Build history of the part. All positions in model axes, mm. Face numbers are marked on the shaded views. A direction names the side the tool comes from. Coordinates: 2 decimals unless noted, no trailing zeros. Order: outer loops, then holes, each group sorted by start corner. A loop starts at its lowest first (then second) coordinate and runs counter-clockwise, first axis right, second up. Notation, with made-up numbers: M 41.5,76 L 72.5,76 A27 cw 72.5,97 Z; hole C 60.5,-29 d10. An arc over 180 degrees is marked long. Write item = value, one per line. Start each with the question number.
Q1. Band-saw the part on D-D on x = 41.5. Write the cut outline in (y, z).
Q2. Band-saw the part on A-A on y = 18. Write the cut outline in (x, z).
Q3. Pull direction X, two halves, no side cores. Call the marked faces 1, 2, 3 and 4: released by +X, released by -X, zero draft, split by the parting line, or undercut.
Q4. Pin check, flat tips, straight feed: P1, Ø3, axis at x = 68.5, z = 4, coming from the +Y side; P2, Ø3.5, axis at x = 66.91, y = 18, coming from the +Z side; P3, Ø1, axis at x = 72, z = 9, coming from the -Y side; P4, Ø1.6, axis at y = 2.5, z = 4, coming from the +X side. Stop position of each tip, or through.
Q5. 3-axis set-ups, long thin cutter, end or side, ignore diameter. For the marked faces 5 and 6: which of +Z, -Z, +X, -X, +Y, -Y reach the whole face in a straight line?
Q6. Band-saw the part on B-B on x = 71.5. Write the cut outline in (y, z).
Q7. Drill centre lines: probe 1 along X at (y, z) = (17, 2.25); probe 2 along X at (y, z) = (40, 8.5); probe 3 along X at (y, z) = (19.5, 1.5). Where is each one in solid material? Low to high.
Q8. Band-saw the part on C-C on z = 4.25. State how many separate pieces and enclosed holes the cut face has, plus the area to 3 significant figures.
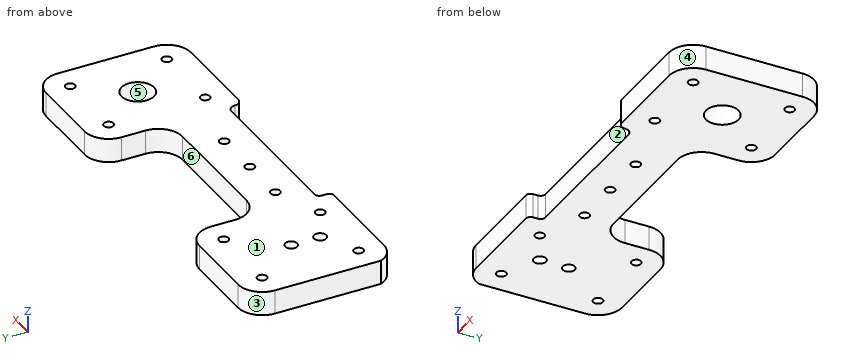
```python
from build123d import *

# Parameters (mm, degrees)
MODEL_R             = 2
MODEL_R_2           = 2.5
MODEL_R_3           = 6.75
MODEL_R_4           = 2.55
BOSS_EXTRUDE1_DEPTH = 10


with BuildPart() as part:
    # Model → Boss-Extrude1 (new body)
    with BuildSketch(Plane.XY):
        with BuildLine():
            Line((-13.089430894, 50), (-13.089430894, 6))
            ThreePointArc((-13.089430894, 6), (-9.401505079, 1.633399735), (-3.924279504, 0))
            Line((-3.924279504, 0), (34.910569106, 0))
            ThreePointArc((34.910569106, 0), (36.324782668, 0.585786438), (36.910569106, 2))
            Line((36.910569106, 2), (36.910569106, 4))
            ThreePointArc((36.910569106, 4), (37.496355543, 5.414213562), (38.910569106, 6))
            Line((38.910569106, 6), (103.910569106, 6))
            ThreePointArc((103.910569106, 6), (106.031889449, 5.121320344), (106.910569106, 3))
            ThreePointArc((106.910569106, 3), (107.789248762, 0.878679656), (109.910569106, 0))
            Line((109.910569106, 0), (146.910569106, 0))
            ThreePointArc((146.910569106, 0), (153.981636918, 2.928932188), (156.910569106, 10))
            Line((156.910569106, 10), (156.910569106, 50))
            ThreePointArc((156.910569106, 50), (153.981636918, 57.071067812), (146.910569106, 60))
            Line((146.910569106, 60), (116.910569106, 60))
            ThreePointArc((116.910569106, 60), (109.839501294, 57.071067812), (106.910569106, 50))
            Line((106.910569106, 50), (106.910569106, 40))
            ThreePointArc((106.910569106, 40), (103.981636918, 32.928932188), (96.910569106, 30))
            Line((96.910569106, 30), (46.910569106, 30))
            ThreePointArc((46.910569106, 30), (39.839501294, 32.928932188), (36.910569106, 40))
            Line((36.910569106, 40), (36.910569106, 50))
            ThreePointArc((36.910569106, 50), (33.981636918, 57.071067812), (26.910569106, 60))
            Line((26.910569106, 60), (-3.089430894, 60))
            ThreePointArc((-3.089430894, 60), (-10.160498706, 57.071067812), (-13.089430894, 50))
        make_face()
        with Locations((26.910569106, 50)):
            Circle(MODEL_R, mode=Mode.SUBTRACT)
        with Locations((26.910569106, 10)):
            Circle(MODEL_R, mode=Mode.SUBTRACT)
        with Locations((11.910569106, 30)):
            Circle(MODEL_R_2, mode=Mode.SUBTRACT)
        with Locations((131.910569106, 30)):
            Circle(MODEL_R_3, mode=Mode.SUBTRACT)
        with Locations((146.910569106, 50)):
            Circle(MODEL_R, mode=Mode.SUBTRACT)
        with Locations((86.910569106, 18)):
            Circle(MODEL_R, mode=Mode.SUBTRACT)
        with Locations((146.910569106, 10)):
            Circle(MODEL_R, mode=Mode.SUBTRACT)
        with Locations((116.910569106, 10)):
            Circle(MODEL_R, mode=Mode.SUBTRACT)
        with Locations((46.910569106, 18)):
            Circle(MODEL_R, mode=Mode.SUBTRACT)
        with Locations((66.910569106, 18)):
            Circle(MODEL_R, mode=Mode.SUBTRACT)
        with Locations((116.910569106, 50)):
            Circle(MODEL_R, mode=Mode.SUBTRACT)
        with Locations((11.910569106, 18)):
            Circle(MODEL_R_4, mode=Mode.SUBTRACT)
        with Locations((-3.089430894, 10)):
            Circle(MODEL_R, mode=Mode.SUBTRACT)
        with Locations((-3.089430894, 50)):
            Circle(MODEL_R, mode=Mode.SUBTRACT)
    extrude(amount=BOSS_EXTRUDE1_DEPTH)


solid = part.part
```
Recorded:
q1.outline = M 6,0 L 31.59,0 L 31.59,10 L 6,10 Z
q2.outline = M -13.09,0 L 9.36,0 L 9.36,10 L -13.09,10 Z; M 14.46,0 L 44.91,0 L 44.91,10 L 14.46,10 Z; M 48.91,0 L 64.91,0 L 64.91,10 L 48.91,10 Z; M 68.91,0 L 84.91,0 L 84.91,10 L 68.91,10 Z; M 88.91,0 L 156.91,0 L 156.91,10 L 88.91,10 Z
q3.face_1 = zero draft
q3.face_2 = undercut
q3.face_3 = released by -X
q3.face_4 = released by +X
q4.P1 = 30
q4.P2 = through
q4.P3 = 6
q4.P4 = 154.33
q5.face_5 = +Z, -Z
q5.face_6 = +Z, -Z, +Y
q6.outline = M 6,0 L 30,0 L 30,10 L 6,10 Z
q7.probe_1 = -13.09 to 9.56, 14.26 to 45.18, 48.64 to 65.18, 68.64 to 85.18, 88.64 to 156.91
q7.probe_2 = -13.09 to 36.91, 106.91 to 156.91
q7.probe_3 = -13.09 to 9.85, 13.97 to 45.59, 48.23 to 65.59, 68.23 to 85.59, 88.23 to 156.91
q8.separate_pieces = 1
q8.enclosed_holes = 14
q8.area = 7,280 mm2
